Build history of the part. All positions in model axes, mm. A direction names the side the tool comes from. Round coordinates to 2 decimals unless told otherwise and drop trailing zeros. Write each loop counter-clockwise with the first axis right and the second up, starting at its lowest first coordinate (ties: lowest second). Pieces come first, ordered by that corner, then holes.
1) Wall check: probe 1 along Y at (x, z) = (20, 17); probe 2 along X at (y, z) = (-309.5, 16); probe 3 along Z at (x, y) = (74.5, -248). Give the ranges that are in metal, low to high.
2) Flat gauge pins, fed straight in: pin 1 (4 mm diameter, centred on x = 167.5, y = -96, fed in from +Z); pin 2 (1.8 mm diameter, centred on x = 50.5, z = 15, fed in from +Y); pin 3 (8 mm diameter, centred on y = -95.5, z = 17, fed in from -X). Where does each tip first touch, or does it go through?
3) Saw through at B-B (x = 210). Write the cut outline in (y, z) (3 decimals), plus the area to 3 significant figures.
4) Pull direction X, two halves, no side cores. Call faces 4 (the flat face through (194, -302, 21)), 5 (the cylindrical face through (50.704, -300.517, 16.479)), 6 (the flat face through (47.5, -301, 14)): +X half, -X half, draft (parallel to the pull), parting line (faces both ways), or undercut.
5) Which spindle directions (+Z, -Z, +X, -X, +Y, -Y) get a long thin tool onto all of the face, cutting with end or side? Do faces 1 (the flat face through (168.001, -235, 12)), 2 (the flat face through (18.5, -302, 21)), 3 (the flat face through (54, -33, 21)). Say none if no direction does.
6) Saw through at A-A (y = -273). Write the cut outline in (x, z), plus the area to 3 significant figures.
from build123d import *

# Parameters (mm, degrees)
SKETCH1_W               = 228.6
SKETCH1_H               = 339.725
BOSS_EXTRUDE1_DEPTH     = 6
SKETCH2_W               = 6.5
SKETCH2_H               = 20
BOSS_EXTRUDE2_DEPTH     = 24
SKETCH3_R               = 4
CUT_EXTRUDE1_DEPTH      = 19.5
CUT_EXTRUDE1_DEPTH_BACK = 211.1
FILLET2_R               = 5


with BuildPart() as part:
    # Sketch1 → Boss-Extrude1 (new body)
    with BuildSketch(Plane.XY):
        with Locations((114.3, -169.8625)):
            Rectangle(SKETCH1_W, SKETCH1_H)
    extrude(amount=BOSS_EXTRUDE1_DEPTH)

    # Sketch2 → Boss-Extrude2 (add)
    with BuildSketch(Plane.XY.offset(6)):
        with Locations((21.75, -35.2425)):
            Rectangle(SKETCH2_W, SKETCH2_H)
        with Locations((50.75, -35.2425)):
            Rectangle(SKETCH2_W, SKETCH2_H)
        with Locations((190.75, -35.2425)):
            Rectangle(SKETCH2_W, SKETCH2_H)
        with Locations((161.75, -35.2425)):
            Rectangle(SKETCH2_W, SKETCH2_H)
        with Locations((133.75086248, -104.5325)):
            Rectangle(SKETCH2_W, SKETCH2_H)
        with Locations((164.75086248, -104.5325)):
            Rectangle(SKETCH2_W, SKETCH2_H)
        with Locations((164.75086248, -235.1925)):
            Rectangle(SKETCH2_W, SKETCH2_H)
        with Locations((21.75, -304.4825)):
            Rectangle(SKETCH2_W, SKETCH2_H)
        with Locations((50.75, -304.4825)):
            Rectangle(SKETCH2_W, SKETCH2_H)
        with Locations((190.75, -304.4825)):
            Rectangle(SKETCH2_W, SKETCH2_H)
        with Locations((161.75, -304.4825)):
            Rectangle(SKETCH2_W, SKETCH2_H)
        with Locations((133.75086248, -235.1925)):
            Rectangle(SKETCH2_W, SKETCH2_H)
    extrude(amount=BOSS_EXTRUDE2_DEPTH)

    # Sketch3 → Cut-Extrude1 (cut, two sides)
    with BuildSketch(Plane.ZY.offset(-18.5)) as cut_extrude1_sk:
        with Locations((17, -35.2425)):
            Circle(SKETCH3_R)
        with Locations((17, -235.1925)):
            Circle(SKETCH3_R)
        with Locations((17, -304.4825)):
            Circle(SKETCH3_R)
        with Locations((17, -104.5325)):
            Circle(SKETCH3_R)
        with BuildLine():
            Line((17, -25.2425), (17, -12.982943413))
            Line((17, -12.982943413), (50.949532367, -12.982943413))
            Line((50.949532367, -12.982943413), (50.949532367, -57.481006387))
            Line((50.949532367, -57.481006387), (17, -57.481006387))
            Line((17, -57.481006387), (17, -45.2425))
            ThreePointArc((17, -45.2425), (27, -35.2425), (17, -25.2425))
        make_face()
        with BuildLine():
            Line((51.442304634, -132.399123951), (17, -132.399123951))
            Line((17, -132.399123951), (17, -114.5325))
            ThreePointArc((17, -114.5325), (27, -104.5325), (17, -94.5325))
            Line((17, -94.5325), (17, -71.59149594))
            Line((17, -71.59149594), (51.442304634, -71.59149594))
            Line((51.442304634, -71.59149594), (51.442304634, -132.399123951))
        make_face()
        with BuildLine():
            Line((51.599532243, -270.375386727), (17, -270.375386727))
            Line((17, -270.375386727), (17, -245.1925))
            ThreePointArc((17, -245.1925), (27, -235.1925), (17, -225.1925))
            Line((17, -225.1925), (17, -207.306351849))
            Line((17, -207.306351849), (51.599532243, -207.306351849))
            Line((51.599532243, -207.306351849), (51.599532243, -270.375386727))
        make_face()
        with BuildLine():
            Line((51.621034016, -326.721115515), (17, -326.721115515))
            Line((17, -326.721115515), (17, -314.4825))
            ThreePointArc((17, -314.4825), (27, -304.4825), (17, -294.4825))
            Line((17, -294.4825), (17, -282.222834285))
            Line((17, -282.222834285), (51.621034016, -282.222834285))
            Line((51.621034016, -282.222834285), (51.621034016, -326.721115515))
        make_face()
    extrude(amount=CUT_EXTRUDE1_DEPTH, mode=Mode.SUBTRACT)
    extrude(cut_extrude1_sk.sketch, amount=-CUT_EXTRUDE1_DEPTH_BACK, mode=Mode.SUBTRACT)

    # Fillet2
    fillet2_edges = [part.edges().sort_by_distance(p)[0] for p in [
        (190.75, -45.2425, 6),
        (194, -35.2425, 6),
        (190.75, -25.2425, 6),
        (50.75, -45.2425, 6),
        (54, -35.2425, 6),
        (50.75, -25.2425, 6),
        (21.75, -25.2425, 6),
        (18.5, -35.2425, 6),
        (21.75, -45.2425, 6),
        (161.75, -25.2425, 6),
        (158.5, -35.2425, 6),
        (161.75, -45.2425, 6),
        (161.75, -294.4825, 6),
        (161.75, -314.4825, 6),
        (158.5, -304.4825, 6),
        (190.75, -314.4825, 6),
        (194, -304.4825, 6),
        (190.75, -294.4825, 6),
        (50.75, -314.4825, 6),
        (54, -304.4825, 6),
        (50.75, -294.4825, 6),
        (21.75, -294.4825, 6),
        (21.75, -314.4825, 6),
        (18.5, -304.4825, 6),
        (164.75086248, -114.5325, 6),
        (164.75086248, -94.5325, 6),
        (168.00086248, -104.5325, 6),
        (133.75086248, -94.5325, 6),
        (130.50086248, -104.5325, 6),
        (133.75086248, -114.5325, 6),
    ]]
    fillet(fillet2_edges, radius=FILLET2_R)


solid = part.part
Evaluation:
1. probe 1: y = -314.48 to -308.48, -300.48 to -294.48, -45.24 to -39.24, -31.24 to -25.24
1. probe 2: x = 18.5 to 25, 47.5 to 54, 158.5 to 165, 187.5 to 194
1. probe 3: z = 0 to 6
2. pin 1: stops at z = 24.57
2. pin 2: stops at y = -25.24
2. pin 3: stops at x = 130.5
3. outline: (-339.725, 0) - (0, 0) - (0, 6) - (-339.725, 6) - close
3. area: 2,040 mm2
4. face 4: +X half
4. face 5: draft
4. face 6: undercut
5. face 1: +Z, +X, -Y
5. face 2: +Z, -X, +Y, -Y
5. face 3: +Z, +Y, -Y
6. outline: (0, 0) - (228.6, 0) - (228.6, 6) - (0, 6) - close
6. area: 1,370 mm2
